Autodesk Inventor part; units mm, degrees
ref_plane "YZ Plane" through (0, 0, 0) normal (1, 0, 0) x (0, 1, 0)
ref_plane "XZ Plane" through (0, 0, 0) normal (0, 1, 0) x (-1, 0, 0)
ref_plane "XY Plane" through (0, 0, 0) normal (0, 0, 1) x (1, 0, 0)
sketch "Sketch1" plane through (0, 0, 0) normal (0, 0, 1) x (1, 0, 0)
  line L0 (-19, 19) -> (19, 19)
  line L1 (19, 19) -> (19, -19)
  line L2 (19, -19) -> (-19, -19)
  line L3 (-19, -19) -> (-19, 19)
  line L4 (-19, 19) -> (19, -19) construction
  line L5 (19, 19) -> (-19, -19) construction
  circle A0 centre (0, 0) radius 4.5
  dimension "d0" = 38
  dimension "d1" = 38
  dimension "d2" = 9
extrude "Extrusion1" add sketch "Sketch1" along normal mid plane 11.64
sketch "Sketch4" plane through (0, 0, 5.82) normal (0, 0, 1) x (1, 0, 0)
  line L0 (-11.25, -11.25) -> (11.25, -11.25) construction
  line L1 (11.25, -11.25) -> (11.25, 11.25) construction
  line L2 (11.25, 11.25) -> (-11.25, 11.25) construction
  line L3 (-11.25, 11.25) -> (-11.25, -11.25) construction
  line L4 (-11.25, -11.25) -> (11.25, 11.25) construction
  line L5 (11.25, -11.25) -> (-11.25, 11.25) construction
  point P0 (0, 0)
  point P1 (-7, -7)
  point P2 (0, 0)
  point P3 (0, 0)
  point P4 (-7, 7)
  point P5 (7, -7)
  point P6 (7, 7)
  dimension "d17" = 22.5
  dimension "d18" = 22.5
  dimension "d47" = 7
  dimension "d48" = 7
  dimension "d51" = 14
  dimension "d54" = 14
sketch "Sketch5" plane through (0, 0, -5.82) normal (0, 0, -1) x (-1, 0, 0)
  circle A0 centre (0, 0) radius 4.5
  circle A1 centre (0, 0) radius 15.24
  dimension "d19" = 30.48
extrude "Extrusion2" cut sketch "Sketch5" against normal blind 8.64 contours A0 | A1
sketch "Sketch6" plane through (-19, 19, 5.82) normal (0, 1, 0) x (1, 0, 0)
  line L0 (0, 11.64) -> (38, 11.64)
  line L1 (3.76, 3) -> (34.24, 3)
  line L2 (10, 11.64) -> (28, 11.64)
  line L3 (28, 11.64) -> (28, 3)
  line L4 (28, 3) -> (10, 3)
  line L5 (10, 3) -> (10, 11.64)
  line L6 (0, 11.64) -> (0, 0)
  line L7 (38, 11.64) -> (38, 0)
  point P0 (19, 5.82)
  point P1 (10, 3)
  dimension "d22" = 10
  dimension "d23" = 10
extrude "Extrusion3" cut sketch "Sketch6" against normal through all
sketch "Sketch7" plane through (19, -19, 5.82) normal (1, 0, 0) x (0, 0, -1)
  line L0 (11.64, 31.2987) -> (11.64, 6.7013)
  line L1 (3, 31.2987) -> (3, 6.7013)
  line L2 (11.64, 28) -> (3, 28)
  line L3 (3, 28) -> (3, 10)
  line L4 (3, 10) -> (11.64, 10)
  line L5 (11.64, 10) -> (11.64, 28)
  line L6 (11.64, 38) -> (0, 38)
  line L7 (11.64, 0) -> (0, 0)
  point P0 (5.82, 19)
  point P1 (11.64, 10)
  point P2 (3, 28)
  dimension "d26" = 10
  dimension "d27" = 10
extrude "Extrusion4" cut sketch "Sketch7" against normal through all
sketch "Sketch8" plane through (0, 0, -5.82) normal (0, 0, -1) x (-1, 0, 0)
  line L0 (-12.2987, -9) -> (-19, -9)
  line L1 (-19, -9) -> (-19, -19)
  line L2 (-19, -19) -> (-9, -19)
  line L3 (-9, -19) -> (-9, -12.2987)
  arc A0 (-12.2987, -9) -> (-9, -12.2987) centre (0, 0) ccw
  point P0 (-15, -15)
  point P1 (-15, 15)
  point P2 (15, -15)
  point P3 (15, 15)
  dimension "d30" = 15
  dimension "d31" = 15
  dimension "d34" = 30
  dimension "d37" = 30
hole "Hole1" at (15, -15, -5.82) at (15, 15, -5.82) at (-15, 15, -5.82) at (-15, -15, -5.82) direction (0, 0, 1) diameter 3.242 depth 4
hole "Hole2" at (-7, -7, 5.82) at (-7, 7, 5.82) at (7, -7, 5.82) at (7, 7, 5.82) direction (0, 0, -1) diameter 1.567 end through all
sketch "Sketch9" plane through (0, 0, 5.82) normal (0, 0, 1) x (1, 0, 0)
  circle A0 centre (15, -15) radius 1.621
  circle A1 centre (-15, -15) radius 1.621
  circle A2 centre (-15, 15) radius 1.621
  circle A3 centre (15, 15) radius 1.621
  point P0 (0, 0)
hole "Hole3" at (15, -15, 5.82) at (-15, -15, 5.82) at (-15, 15, 5.82) at (15, 15, 5.82) direction (0, 0, -1) diameter 3.242 depth 5
equation "\"d1\" = d0"
equation "\"d18\" = d17"
properties part number "pmtbase"
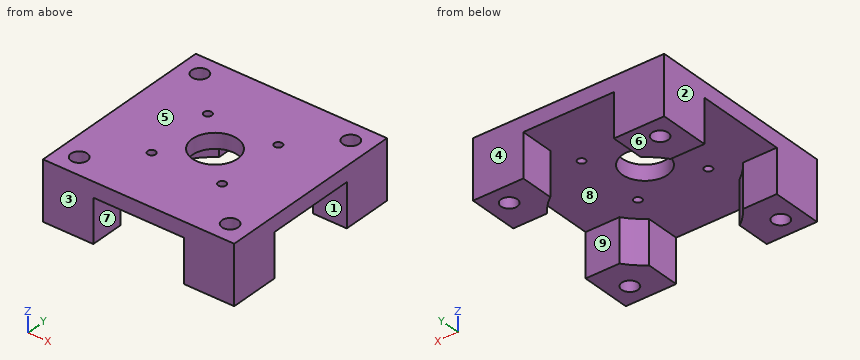
The listing builds one solid part. Answer for the finished solid, in the listing's coordinates (mm). Face numbers are marked on the shaded views. A direction names the side the tool comes from. Give positions to 0.01 mm unless a question says otherwise; leave off trailing zeros. Order: outer loops, then holes, each group sorted by start corner. A loop starts at its lowest first (then second) coordinate and runs counter-clockwise, first axis right, second up. Notation, with made-up numbers: (83, 57) -> (96, 57) arc R14 ccw to (96, 74) -> close; hole circle Ø5 at (78.5, 60). An arc over 180 degrees is marked (long way). One line per item, written item: value.
1) Flat-ended cylindrical pins translate along their axes: P1, Ø1.6, axis at x = -14.5, y = 15, coming from the -Z side; P2, Ø1.8, axis at x = 7, y = 7, coming from the -Z side; P3, Ø1, axis at x = 15, y = -14, coming from the +Z side; P4, Ø0.9, axis at x = -7, y = -7, coming from the +Z side. Find the tip coordinate at first contact, or state that the pin passes through.
Reported:
P1: stops at z = -1.82
P2: stops at z = 2.82
P3: stops at z = 0.82
P4: passes through
2) Determine the mould class of the marked faces 1, 2, 3 and 4 for opening direction Y: pulls with the +Y half, pulls with the -Y half, needs draft (parallel to the pull), parting line crosses it, or undercut.
Reported:
face 1: undercut
face 2: needs draft
face 3: pulls with the -Y half
face 4: pulls with the +Y half
3) Find the intervals of material crossed by line 1 (X direction, y = -7, z = 4.75); line 2 (Y direction, x = 15, z = 2.35), in increasing order.
Reported:
line 1: x = -19 to -7.78, -6.22 to 6.22, 7.78 to 19
line 2: y = -19 to -16.62, -13.38 to -9, 9 to 13.38, 16.62 to 19
4) Find section A-A, the plane z = -3.5. Determine the outline of the cut face in (x, y).
Reported:
outline: (-19, -19) -> (-9, -19) -> (-9, -12.3) arc R15.24 cw to (-12.3, -9) -> (-19, -9) -> close; (-19, 9) -> (-12.3, 9) arc R15.24 cw to (-9, 12.3) -> (-9, 19) -> (-19, 19) -> close; (9, -19) -> (19, -19) -> (19, -9) -> (12.3, -9) arc R15.24 cw to (9, -12.3) -> close; (9, 12.3) arc R15.24 cw to (12.3, 9) -> (19, 9) -> (19, 19) -> (9, 19) -> close; hole circle Ø3.24 at (-15, -15); hole circle Ø3.24 at (-15, 15); hole circle Ø3.24 at (15, -15); hole circle Ø3.24 at (15, 15)
5) A tool of negligible diameter and unlimited length cuts with its end or side. For the marked faces 5, 6, 7, 8 and 9, from which of +Z, -Z, +X, -X, +Y, -Y can it reach the whole face along a straight path? Write none if from no direction.
Reported:
face 5: +Z, +X, -X, +Y, -Y
face 6: -Z, +X, -X, +Y, -Y
face 7: -Z, +Y, -Y
face 8: -Z
face 9: -Z, +X, -X
6) Find section C-C, the plane y = 0. Determine the outline of the cut face in (x, z).
Reported:
outline: (-19, 2.82) -> (-4.5, 2.82) -> (-4.5, 5.82) -> (-19, 5.82) -> close; (4.5, 2.82) -> (19, 2.82) -> (19, 5.82) -> (4.5, 5.82) -> close
7) Find section B-B, the plane x = 7. Determine the outline of the cut face in (y, z), plus the area to 3 significant figures.
Reported:
outline: (-19, 2.82) -> (-7.78, 2.82) -> (-7.78, 5.82) -> (-19, 5.82) -> close; (-6.22, 2.82) -> (6.22, 2.82) -> (6.22, 5.82) -> (-6.22, 5.82) -> close; (7.78, 2.82) -> (19, 2.82) -> (19, 5.82) -> (7.78, 5.82) -> close
area: 105 mm^2
